Here's how the part is built. I have some questions about the finished solid (model axes, mm). A direction names the side the tool comes from. Round coordinates to 2 decimals unless told otherwise and drop trailing zeros. Write each loop counter-clockwise with the first axis right and the second up, starting at its lowest first coordinate (ties: lowest second). Pieces come first, ordered by that corner, then holes. Notation, with made-up numbers: (47.25, -26) -> (90.25, -26) arc R19 cw to (90.25, -9) -> close; hole circle Ø4 at (24.25, 67.25). An arc over 180 degrees is marked (long way). Answer in a Markdown table with one row per item.
Autodesk Inventor part; units mm, degrees
ref_plane "YZ Plane" through (0, 0, 0) normal (1, 0, 0) x (0, 1, 0)
ref_plane "XZ Plane" through (0, 0, 0) normal (0, 1, 0) x (-1, 0, 0)
ref_plane "XY Plane" through (0, 0, 0) normal (0, 0, 1) x (1, 0, 0)
sketch "スケッチ1" plane through (0, 0, 0) normal (0, 0, 1) x (1, 0, 0)
  circle A0 centre (0, 0) radius 1.5
  dimension "d0" = 3
extrude "押し出し1" add sketch "スケッチ1" along normal blind 6
sketch "スケッチ2" plane through (0, 0, 6) normal (0, 0, 1) x (1, 0, 0)
  circle A0 centre (0, 0) radius 1.5
  circle A1 centre (0, 0) radius 3
  dimension "d3" = 6
extrude "押し出し2" add sketch "スケッチ2" along normal blind 2 contours A0 | A1
fillet "フィレット1" radius 2 1 edges at (-3, 0, 8)
thread "ねじ1"
sketch "スケッチ3" plane through (0, 0, 0) normal (0, 0, -1) x (-1, 0, 0)
  circle A0 centre (0, 0) radius 1.5
extrude "押し出し3" add sketch "スケッチ3" along normal blind 9
sketch "スケッチ4" plane through (0, 0, -9) normal (0, 0, -1) x (-1, 0, 0)
  circle A0 centre (0, 0) radius 1.5
extrude "押し出し4" add sketch "スケッチ4" along normal blind 20
properties part number "SB　35mmなべネジ" material "Steel, Mild"
1) I want a section at A-A, the plane z = -10.5. List the corners of the cut face in (x, y) for me.
Response:
| item | result |
|---|---|
| outline | circle Ø3 at (0, 0) |
2) For pin 1 (3 mm diameter, centred on y = 1, z = -18.5, fed in from +X); pin 2 (2 mm diameter, centred on y = 1.5, z = -4.5, fed in from +X); pin 3 (2 mm diameter, centred on x = -2.5, y = 1, fed in from -Z), each with a flat end and sliding along its axis, tell me the tip position at first contact or that it passes through.
Response:
| item | result |
|---|---|
| pin 1 | stops at x = 1.5 |
| pin 2 | stops at x = 1.41 |
| pin 3 | stops at z = 6 |
3) Which directions (+Z, -Z, +X, -X, +Y, -Y) give clear straight access to the entire face, cutting with the end or side of a thin tool? Please do faces 1 (the face through (1.3, -1.3, 6)), 2 (the face through (0, 0, -29)).
Response:
| item | result |
|---|---|
| face 1 | -Z |
| face 2 | -Z, +X, -X, +Y, -Y |
4) I need wall thicknesses on line 1 (Y direction, x = 0, z = -2.5); line 2 (Z direction, x = 2, y = 0.5); line 3 (Z direction, x = -2, y = 1.75). Which ranges of each line are inside material? Lowest first, please. Write a range as [from, to].
Response:
| item | result |
|---|---|
| line 1 | y = [-1.5, 1.5] |
| line 2 | z = [6, 7.7] |
| line 3 | z = [6, 7.12] |
